Work out the finished part from the listing and answer in its coordinate system (mm). Coordinates: 2 decimals unless noted, no trailing zeros. Loops run counter-clockwise (first coordinate to the right, second up) from the corner with the lowest first, then second, coordinate; pieces in that order, holes last. Notation, with made-up numbers: (7, -17) -> (39, -17) arc R20 cw to (39, 18) -> close; hole circle Ø3 at (12, 65.25). An arc over 180 degrees is marked (long way). Use a Markdown table: item, result.
from build123d import *

# Parameters (mm, degrees)
SKETCH1_W           = 30
SKETCH1_H           = 220
SKETCH1_R           = 3.1
BOSS_EXTRUDE1_DEPTH = 12
FILLET1_R           = 5


with BuildPart() as part:
    # Sketch1 → Boss-Extrude1 (new body)
    with BuildSketch(Plane(origin=(0, 0, 0), x_dir=(0, 0, -1), z_dir=(1, 0, 0))):
        with Locations((0, 95)):
            Rectangle(SKETCH1_W, SKETCH1_H)
        Circle(SKETCH1_R, mode=Mode.SUBTRACT)
        with Locations((0, 20)):
            Circle(SKETCH1_R, mode=Mode.SUBTRACT)
        with Locations((0, 120)):
            Circle(SKETCH1_R, mode=Mode.SUBTRACT)
        with Locations((0, 190)):
            Circle(SKETCH1_R, mode=Mode.SUBTRACT)
    extrude(amount=BOSS_EXTRUDE1_DEPTH)

    # Fillet1
    fillet1_edges = [part.edges().sort_by_distance(p)[0] for p in [
        (6, 205, 15),
        (6, 205, -15),
        (6, -15, -15),
        (6, -15, 15),
    ]]
    fillet(fillet1_edges, radius=FILLET1_R)


solid = part.part
Q1. Given pin 1 Ø5 at (y, z) = (0, 0) entering from -X, flat-ended and moving along its own axis, determine where the tip first touches the part or whether it passes through.
Solved:
| item | result |
|---|---|
| pin 1 | through |
Q2. Section A-A on z = 0 is taken. Determine the outline of the cut face in (x, y).
Solved:
| item | result |
|---|---|
| outline | (0, -15) -> (12, -15) -> (12, -3.1) -> (0, -3.1) -> close; (0, 3.1) -> (12, 3.1) -> (12, 16.9) -> (0, 16.9) -> close; (0, 23.1) -> (12, 23.1) -> (12, 116.9) -> (0, 116.9) -> close; (0, 123.1) -> (12, 123.1) -> (12, 186.9) -> (0, 186.9) -> close; (0, 193.1) -> (12, 193.1) -> (12, 205) -> (0, 205) -> close |
Q3. Section B-B on y = 0 is taken. Determine the outline of the cut face in (x, z), and give its area (3 significant figures).
Solved:
| item | result |
|---|---|
| outline | (0, -15) -> (12, -15) -> (12, -3.1) -> (0, -3.1) -> close; (0, 3.1) -> (12, 3.1) -> (12, 15) -> (0, 15) -> close |
| area | 286 mm² |
Q4. Section C-C on x = 8.5 is taken. Determine the outline of the cut face in (y, z), and give its area (3 significant figures).
Solved:
| item | result |
|---|---|
| outline | (-15, -10) arc R5 ccw to (-10, -15) -> (200, -15) arc R5 ccw to (205, -10) -> (205, 10) arc R5 ccw to (200, 15) -> (-10, 15) arc R5 ccw to (-15, 10) -> close; hole circle Ø6.2 at (0, 0); hole circle Ø6.2 at (20, 0); hole circle Ø6.2 at (120, 0); hole circle Ø6.2 at (190, 0) |
| area | 6,460 mm² |
Q5. Consider line 1 (Y direction, x = 5.25, z = 0); line 2 (Z direction, x = 6.75, y = 190); line 3 (Z direction, x = 5, y = 121). Determine where each line is inside the solid, lowest interval first. Write a range as [from, to].
Solved:
| item | result |
|---|---|
| line 1 | [-15, -3.1], [3.1, 16.9], [23.1, 116.9], [123.1, 186.9], [193.1, 205] |
| line 2 | [-15, -3.1], [3.1, 15] |
| line 3 | [-15, -2.93], [2.93, 15] |
Q6. Determine the mould class of faces 1 (the flat face through (0, 97, 0)), 2 (the cylindrical face through (5.916, 16.974, 0.672)), 3 (the cylindrical face through (6, 204, -13)) for opening direction Y: pulls with the +Y half, pulls with the -Y half, needs draft (parallel to the pull), parting line crosses it, or undercut.
Solved:
| item | result |
|---|---|
| face 1 | needs draft |
| face 2 | undercut |
| face 3 | pulls with the +Y half |
